```python
from build123d import *

# Parameters (mm, degrees)
F0_W     = 63.5
F0_H     = 31.75
F1_DEPTH = 25.4
F3_DEPTH = 25.4


with BuildPart() as f1:
    # F0 (on Front) → F1 (new body)
    with BuildSketch(Plane.XZ):
        with Locations((31.75, 15.875)):
            Rectangle(F0_W, F0_H)
    extrude(amount=F1_DEPTH)

    # F2 (on face) → F3 (cut)
    with BuildSketch(Plane.XZ.offset(25.4)):
        Polygon((44.45, 31.75), (19.05, 31.75), (31.75, 19.05), align=None)
        Polygon((19.05, 31.75), (6.35, 31.75), (31.75, 6.35), (31.75, 19.05), align=None)
        Polygon((31.75, 19.05), (31.75, 6.35), (57.15, 31.75), (44.45, 31.75), align=None)
    extrude(amount=-F3_DEPTH, mode=Mode.SUBTRACT)


solid = f1.part
```
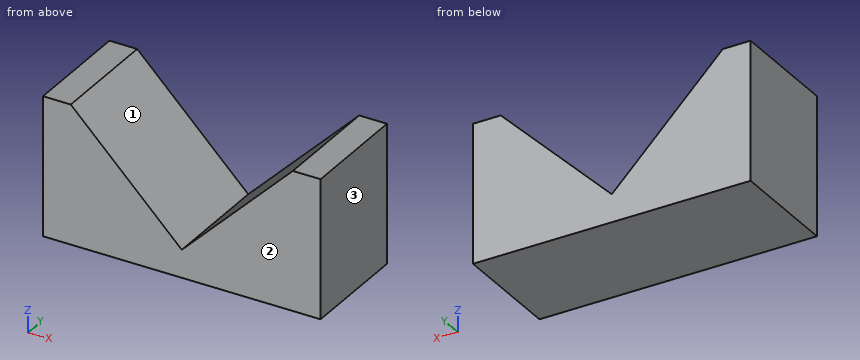
Geometry check sheet. Reference: the model listing, model coordinates, mm. Face numbers are marked on the shaded views. Give positions to 0.01 mm unless a question says otherwise; leave off trailing zeros. Order: outer loops, then holes, each group sorted by start corner. A loop starts at its lowest first (then second) coordinate and runs counter-clockwise, first axis right, second up.
1. Section check A-A, the plane z = 23. Enter the section's corners in (x, y), and give its area (3 significant figures).
2. Section check D-D, the plane x = 15.5. Enter the section's corners in (y, z), and give its area (3 significant figures).
3. Gauge pin test, flat ends, axial feed: pin 1 Ø2 at (x, y) = (37, -19.5) entering from +Z; pin 2 Ø12 at (y, z) = (-13.5, 8) entering from -X. Record the tip position at first contact, or that the pin passes through.
4. Release check for a two-part mould opening along X. For the marked faces 1, 2 and 3 record: pulls with the +X half, pulls with the -X half, needs draft (parallel to the pull), parting line crosses it, or undercut.
5. Section check C-C, the plane z = 17. Enter the section's corners in (x, y), and give its area (3 significant figures).
6. Thickness scan on L1, parallel to X at y = -11.5, z = 6.5; L2, parallel to X at y = -7.5, z = 29.5; L3, parallel to Z at x = 25, y = -2.25. Record the ranges inside material, lowest first.
7. Section check B-B, the plane y = -14.25. Enter the section's corners in (x, z), and give its area (3 significant figures).
Values follow:
1. outline: (0, -25.4) - (15.1, -25.4) - (15.1, 0) - (0, 0) - close; (48.4, -25.4) - (63.5, -25.4) - (63.5, 0) - (48.4, 0) - close
1. area: 767 mm2
2. outline: (-25.4, 0) - (0, 0) - (0, 22.6) - (-25.4, 22.6) - close
2. area: 574 mm2
3. pin 1: stops at z = 12.6
3. pin 2: stops at x = 0
4. face 1: undercut
4. face 2: needs draft
4. face 3: pulls with the +X half
5. outline: (0, -25.4) - (21.1, -25.4) - (21.1, 0) - (0, 0) - close; (42.4, -25.4) - (63.5, -25.4) - (63.5, 0) - (42.4, 0) - close
5. area: 1,070 mm2
6. L1: x = 0 to 31.6, 31.9 to 63.5
6. L2: x = 0 to 8.6, 54.9 to 63.5
6. L3: z = 0 to 13.1
7. outline: (0, 0) - (63.5, 0) - (63.5, 31.75) - (57.15, 31.75) - (31.75, 6.35) - (6.35, 31.75) - (0, 31.75) - close
7. area: 1,370 mm2
